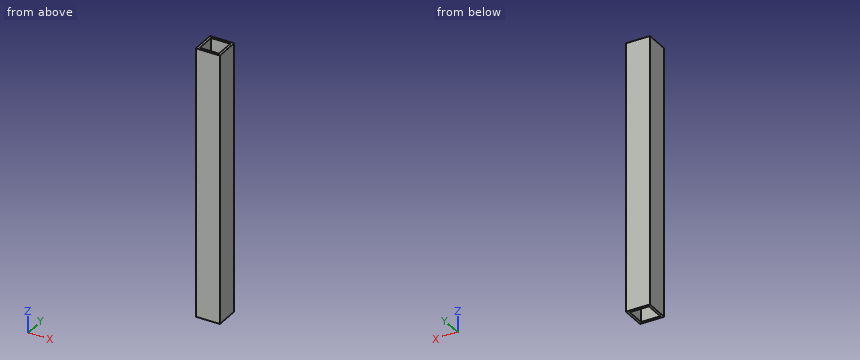
Autodesk Inventor part; units mm, degrees
ref_plane "YZ Plane" through (0, 0, 0) normal (1, 0, 0) x (0, 1, 0)
ref_plane "XZ Plane" through (0, 0, 0) normal (0, 1, 0) x (-1, 0, 0)
ref_plane "XY Plane" through (0, 0, 0) normal (0, 0, 1) x (1, 0, 0)
sketch "Sketch1" plane through (0, 0, 0) normal (0, 0, 1) x (1, 0, 0)
  line L0 (-15.875, 15.875) -> (15.875, 15.875)
  line L1 (15.875, 15.875) -> (15.875, -15.875)
  line L2 (15.875, -15.875) -> (-15.875, -15.875)
  line L3 (-15.875, -15.875) -> (-15.875, 15.875)
  line L4 (12.7, 12.7) -> (-12.7, 12.7)
  line L5 (-12.7, 12.7) -> (-12.7, -12.7)
  line L6 (-12.7, -12.7) -> (12.7, -12.7)
  line L7 (12.7, -12.7) -> (12.7, 12.7)
  point P0 (0, 0)
  point P1 (-15.875, 0)
  point P2 (0, 15.875)
  dimension "d0" = 31.75
  dimension "d1" = 3.175
extrude "Extrusion1" add sketch "Sketch1" along normal mid plane 355.6
properties part number "Handle Slide"
For this review, take the finished solid that the model builds, in its own axes (mm). Coordinates: 2 decimals unless noted, no trailing zeros. Loops run counter-clockwise (first coordinate to the right, second up) from the corner with the lowest first, then second, coordinate; pieces in that order, holes last. Notation, with made-up numbers: (77, -11.75) -> (95, -11.75) arc R30 cw to (95, 10.25) -> close; hole circle Ø3 at (6.5, -30). An arc over 180 degrees is marked (long way). Return JSON: item names as keys, results as strings. Group by question number.
(1) For pin 1 Ø8 at (x, y) = (12, -5) entering from +Z, flat-tipped, find the tip position at first contact; note if it passes through.
(2) Consider section A-A, the plane y = 3. Give the boundary of the cut face in (x, z) (3 decimals), plus the area to 3 significant figures.
(3) To check wall thickness, follow L1, parallel to Y at x = 5, z = -64 (3 decimals). State the ranges of the line that lie inside material, in increasing order.
(4) Consider section C-C, the plane z = -10.5. Give the boundary of the cut face in (x, y) (3 decimals).
Results below:
{
 "1": {"pin 1": "stops at z = 177.8"},
 "2": {"outline": "(-15.875, -177.8) -> (-12.7, -177.8) -> (-12.7, 177.8) -> (-15.875, 177.8) -> close; (12.7, -177.8) -> (15.875, -177.8) -> (15.875, 177.8) -> (12.7, 177.8) -> close", "area": "2,260 mm2"},
 "3": {"L1": "y = -15.875 to -12.7, 12.7 to 15.875"},
 "4": {"outline": "(-15.875, -15.875) -> (15.875, -15.875) -> (15.875, 15.875) -> (-15.875, 15.875) -> close; hole (-12.7, -12.7) -> (12.7, -12.7) -> (12.7, 12.7) -> (-12.7, 12.7) -> close"}
}
